Work out the finished part from the listing and answer in its coordinate system (mm). Round coordinates to 2 decimals unless told otherwise and drop trailing zeros. Answer as a JSON object with one key per item and string values.
```python
from build123d import *

# Parameters (mm, degrees)
SKETCH023_R             = 2.5
PAD006_DEPTH            = 12
SKETCH024_W             = 7
SKETCH024_H             = 6
PAD007_DEPTH            = 4
FILLET005_R             = 1
FILLET006_R             = 1
BODY004_PLACEMENT_ANGLE = 330


with BuildPart() as part:
    # Sketch023 → Pad006 (new body)
    with BuildSketch(Plane.YZ):
        Circle(SKETCH023_R)
    extrude(amount=PAD006_DEPTH)

    # Sketch024 (on Face2 of Pad006) → Pad007 (join)
    with BuildSketch(Plane(origin=(0, 0, 0), x_dir=(0, 1, 0), z_dir=(-1, 0, 0))):
        with Locations((0, 0.5)):
            Rectangle(SKETCH024_W, SKETCH024_H)
    extrude(amount=PAD007_DEPTH)

    # Fillet005
    fillet005_edges = [part.edges().sort_by_distance(p)[0] for p in [
        (-2, 3.5, 2.5),
        (-2, 3.5, -3.5),
        (-2, -3.5, -3.5),
        (-2, -3.5, 2.5),
    ]]
    fillet(fillet005_edges, radius=FILLET005_R)

    # Fillet006
    fillet006_edges = [part.edges().sort_by_distance(p)[0] for p in [
        (12, -2.5, 0),
    ]]
    fillet(fillet006_edges, radius=FILLET006_R)


with BuildPart() as part_1:
    # Body004 placement: moved
    add(part.part.moved(Location((23.239092, -5, -19.251289))).rotate(Axis((23.239092, -5, -19.251289), (0, 1, 0)), BODY004_PLACEMENT_ANGLE))


solid = part_1.part
```
Item 1: Consider line 1 along Y through (x, z) = (26.5, -17.25); line 2 along Z through (x, y) = (24.5, -7); line 3 along Z through (x, y) = (33.25, -2.75). Determine where each line is inside the solid, lowest interval first.
Results found:
{"line 1": "-7.5 to -2.5", "line 2": "-22.56 to -21.44, -20.26 to -16.79", "line 3": "-14.73 to -13.28"}
Item 2: Determine the mould class of faces 1 (the flat face through (33.6, -5, -13.2)), 2 (the flat face through (24.51, -5.83, -21.45)), 3 (the flat face through (22, -8.5, -21)), 4 (the flat face through (23.28, -5.04, -23.27)) for opening direction Z: pulls with the +Z half, pulls with the -Z half, needs draft (parallel to the pull), parting line crosses it, or undercut.
Results found:
{"face 1": "pulls with the +Z half", "face 2": "undercut", "face 3": "needs draft", "face 4": "pulls with the -Z half"}
Item 3: Each of these flat-tipped pins is pushed along its axis until it touches: P1, Ø2, axis at y = -7, z = -17.5, coming from the +X side; P2, Ø2, axis at x = 27, y = -4, coming from the -Z side; P3, Ø4, axis at x = 31, y = -6, coming from the -Z side. Where does it stop, or does it pass through?
Results found:
{"P1": "x = 31.8", "P2": "z = -20.41", "P3": "z = -18.72"}
